Check sheet for the modelled part. Datum: model origin and axes. Units: mm. A direction names the side the tool comes from. Coordinates: 2 decimals unless noted, no trailing zeros. Loops run counter-clockwise (first coordinate to the right, second up) from the corner with the lowest first, then second, coordinate; pieces in that order, holes last.
```python
from build123d import *

# Parameters (mm, degrees)
F0_W     = 630
F0_H     = 911
F0_H_2   = 4
F0_H_3   = 5
F1_DEPTH = 2
F4_DEPTH = 4
F7_DEPTH = 9
F8_W     = 630
F8_H     = 4
F9_DEPTH = 5


with BuildPart() as f1:
    # F0 (on Front) → F1 (new body)
    with BuildSketch(Plane.XZ):
        with Locations((0, -4.5)):
            Rectangle(F0_W, F0_H)
        with Locations((0, 453)):
            Rectangle(F0_W, F0_H_2)
        with Locations((0, 457.5)):
            Rectangle(F0_W, F0_H_3)
    extrude(amount=F1_DEPTH)

    # F6: F4, F5_1 across plane


with BuildPart() as f4:
    # F3 (on offset) → F4 (new body)
    with BuildSketch(Plane.YZ.offset(-315)):
        with BuildLine():
            Line((0, 440), (0, 410))
            Line((0, 410), (14.5, 410))
            ThreePointArc((14.5, 410), (16.6213203436, 410.8786796564), (17.5, 413))
            Line((17.5, 413), (17.5, 425))
            ThreePointArc((17.5, 425), (19.5741329805, 427.4634604283), (22.3549098254, 425.8392852402))
            Line((22.3549098254, 425.8392852402), (27.7746731609, 410.6322336697))
            ThreePointArc((27.7746731609, 410.6322336697), (28.122676008, 410.1739557831), (28.6711867084, 410))
            Line((28.6711867084, 410), (29.0482506613, 410))
            ThreePointArc((29.0482506613, 410), (29.7212390727, 410.2787609273), (30, 410.9517493387))
            Line((30, 410.9517493387), (30, 440))
            Line((30, 440), (0, 440))
        make_face()
    extrude(amount=F4_DEPTH)


with BuildPart() as f5_1:
    # F5: copy of F4
    add(f4.part.moved(Location((0, 0, -700))))


with BuildPart() as f1_1:
    add(f1.part)
    add(f4.part.mirror(Plane.YZ))
    add(f5_1.part.mirror(Plane.YZ))

    # F0 (on Front) → F7 (join)
    with BuildSketch(Plane.XZ):
        with Locations((0, 453)):
            Rectangle(F0_W, F0_H_2)
    extrude(amount=-F7_DEPTH)


    add(f4.part)  # F9 merges F4

    add(f5_1.part)  # F9 merges F5_1
    # F8 (on face) → F9 (join)
    with BuildSketch(Plane.XY.offset(455)):
        with Locations((0, 7)):
            Rectangle(F8_W, F8_H)
    extrude(amount=F9_DEPTH)


solid = f1_1.part
```
1) Set-up check for faces 4 (the flat face through (-311, 15, 425)), 5 (the flat face through (315, -0.3, -70.3)): record each of +Z, -Z, +X, -X, +Y, -Y from which the full face is reachable in a straight line by a thin tool's end or side.
Answer sheet:
face 4: -Z, +Y
face 5: +Z, -Z, +X, +Y, -Y
2) Depth check by flat-ended pin: pin 1 (4 mm diameter, centred on x = -116.5, z = 457, fed in from +Y); pin 2 (4.5 mm diameter, centred on x = 313, y = 10.5, fed in from -Z); pin 3 (3 mm diameter, centred on x = 312, y = 19, fed in from +Z); pin 4 (5 mm diameter, centred on x = -33.5, y = 1.5, fed in from -Z). Enter the tip coordinate at first touch or a pass-through.
Answer sheet:
pin 1: stops at y = 9
pin 2: stops at z = -290
pin 3: stops at z = 440
pin 4: stops at z = -460
3) Section check A-A on x = 71.5. Enter the section's corners in (y, z), plus the area to 3 significant figures.
Answer sheet:
outline: (-2, -460) - (0, -460) - (0, 451) - (9, 451) - (9, 460) - (5, 460) - (5, 455) - (0, 455) - (0, 460) - (-2, 460) - close
area: 1,900 mm2
4) Mould release check, pull along X, two halves, no side actions. Record for faces 1 (the flat face through (-315, -0.3, -70.3)), 2 (the flat face through (-311, 15, -275)), 3 (the flat face through (-4, -2, 6)): +X half, -X half, draft (parallel to the pull), parting line (faces both ways), or undercut.
Answer sheet:
face 1: -X half
face 2: undercut
face 3: draft
5) Section check B-B on z = -35. Enter the section's corners in (x, y), plus the area to 3 significant figures.
Answer sheet:
outline: (-315, -2) - (315, -2) - (315, 0) - (-315, 0) - close
area: 1,260 mm2
6) Scan lines: line 1 (X direction, y = 14.5, z = 414.5); line 2 (Y direction, x = -2, z = -387); line 3 (Z direction, x = 23.5, y = 3). Record each from-to range of solid material in increasing order.
Answer sheet:
line 1: x = -315 to -311, 311 to 315
line 2: y = -2 to 0
line 3: z = 451 to 455
